from build123d import *

# Parameters (mm, degrees)
SKETCH_R  = 1.1
PAD_DEPTH = 6
FILLET_R  = 1


with BuildPart() as part:
    # Sketch → Pad (new body)
    with BuildSketch(Plane.XY):
        with BuildLine():
            ThreePointArc((4.5, 10.5), (0, 15), (-4.5, 10.5))
            Line((-4.5, 10.5), (-4.5, -10.5))
            ThreePointArc((-4.5, -10.5), (0, -15), (4.5, -10.5))
            Line((4.5, -10.5), (4.5, 10.5))
        make_face()
        with Locations((0, 10.5)):
            Circle(SKETCH_R, mode=Mode.SUBTRACT)
        with Locations((0, -10.5)):
            Circle(SKETCH_R, mode=Mode.SUBTRACT)
    extrude(amount=PAD_DEPTH)

    # Fillet
    fillet_edges = [part.edges().sort_by_distance(p)[0] for p in [
        (-4.5, 0, 6),
    ]]
    fillet(fillet_edges, radius=FILLET_R)


solid = part.part
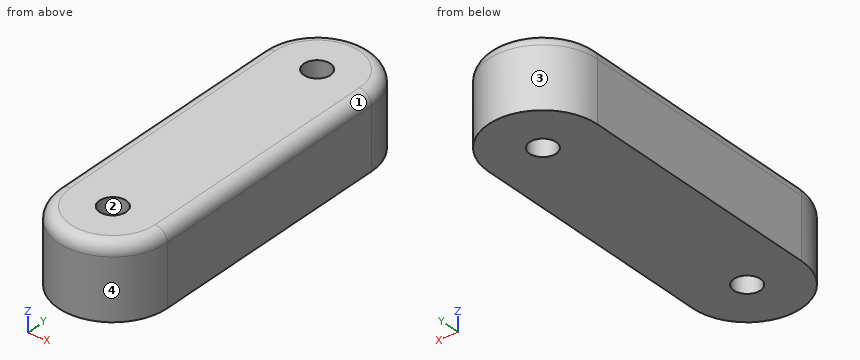
Source: CAD feature listing. Evaluate the final solid. Frame: model axes, mm. Face numbers are marked on the shaded views. Give positions to 0.01 mm unless a question says otherwise; leave off trailing zeros. Write each loop counter-clockwise with the first axis right and the second up, starting at its lowest first coordinate (ties: lowest second). Pieces come first, ordered by that corner, then holes. Notation, with made-up numbers: (-18, 1) -> (4, 1) arc R7 ccw to (4, 12) -> close; hole circle Ø6 at (-21, 78.25). An arc over 180 degrees is marked (long way). Return JSON: item names as keys, results as strings. Group by question number.
1. Mould query, pull axis Y, two halves, no side actions, for the marked faces 1, 2, 3 and 4. Classes: +Y half, -Y half, draft (parallel to the pull), parting line (faces both ways), or undercut.
2. Section A-A, the plane x = 0. Output: boundary loops of the cut face in (y, z).
3. Material intervals for line 1 (Y direction, x = 0, z = 1.4); line 2 (Y direction, x = -1, z = 1.75); line 3 (X direction, y = -11, z = 5.6), sorted ascending. Write a range as from..to.
4. Section B-B, the plane z = 1.5. Output: boundary loops of the cut face in (x, y), then the cut area to 3 significant figures.
5. Pin query (flat end, axial travel): pin 1 Ø1 at (x, z) = (-1, 1.5) entering from +Y. Return the tip coordinate at first contact, or that it passes through.
6. Section C-C, the plane z = 5.5. Output: boundary loops of the cut face in (x, y).
Determined:
{
 "1": {"face 1": "draft", "face 2": "undercut", "face 3": "+Y half", "face 4": "-Y half"},
 "2": {"outline": "(-15, 0) -> (-11.6, 0) -> (-11.6, 6) -> (-14, 6) arc R1 ccw to (-15, 5) -> close; (-9.4, 0) -> (9.4, 0) -> (9.4, 6) -> (-9.4, 6) -> close; (11.6, 0) -> (15, 0) -> (15, 5) arc R1 ccw to (14, 6) -> (11.6, 6) -> close"},
 "3": {"line 1": "y = -15..-11.6, -9.4..9.4, 11.6..15", "line 2": "y = -14.89..-10.96, -10.04..10.04, 10.96..14.89", "line 3": "x = -4.27..-0.98, 0.98..4.27"},
 "4": {"outline": "(-4.5, -10.5) arc R4.5 ccw to (4.5, -10.5) -> (4.5, 10.5) arc R4.5 ccw to (-4.5, 10.5) -> close; hole circle Ø2.2 at (0, -10.5); hole circle Ø2.2 at (0, 10.5)", "area": "245 mm2"},
 "5": {"pin 1": "stops at y = 14.97"},
 "6": {"outline": "(-4.37, -10.5) arc R4.37 ccw to (4.37, -10.5) -> (4.37, 10.5) arc R4.37 ccw to (-4.37, 10.5) -> close; hole circle Ø2.2 at (0, -10.5); hole circle Ø2.2 at (0, 10.5)"}
}
